Source: three-view drawing plus pictorial views. Frame: mm from the lowest corner of the part. Coordinates: 2 decimals unless noted, no trailing zeros. Write each loop counter-clockwise with the first axis right and the second up, starting at its lowest first coordinate (ties: lowest second). Pieces come first, ordered by that corner, then holes. Notation, with made-up numbers: M 69.25,4.5 L 99.25,4.5 A24 ccw 99.25,26.5 Z; hole C -27,87 d4. An arc over 180 degrees is marked long. Write item = value, one per line. Start each with the question number.
Item 1: Ray query, L1, parallel to X at y = 27, z = 9.5; L2, parallel to X at y = 27.5, z = 20.25 (1 decimal); L3, parallel to X at y = 188, z = 11.25. Return the intervals inside material, ascending. Write a range as [from, to].
Item 2: First-contact query: pin 1 Ø10 at (y, z) = (190.5, 13.5) entering from +X (1 decimal); pin 2 Ø5 at (y, z) = (37, 10) entering from -X; pin 3 Ø20 at (x, y) = (265, 30) entering from +Z; pin 4 Ø8 at (y, z) = (38, 13) entering from +X. Flat tips, straight axial feed; report the tip coordinate or a pass-through.
Item 3: Section C-C on y = 188. Output: boundary loops of the cut face in (x, z).
Item 4: Section B-B on z = 4. Output: boundary loops of the cut face in (x, y) (1 decimal), plus the area to 4 significant figures.
Item 5: Section D-D on x = 177. Output: boundary loops of the cut face in (y, z) (1 decimal), plus the area to 3 significant figures.
Item 6: Section A-A on y = 30. Output: boundary loops of the cut face in (x, z), plus the area to 3 significant figures.
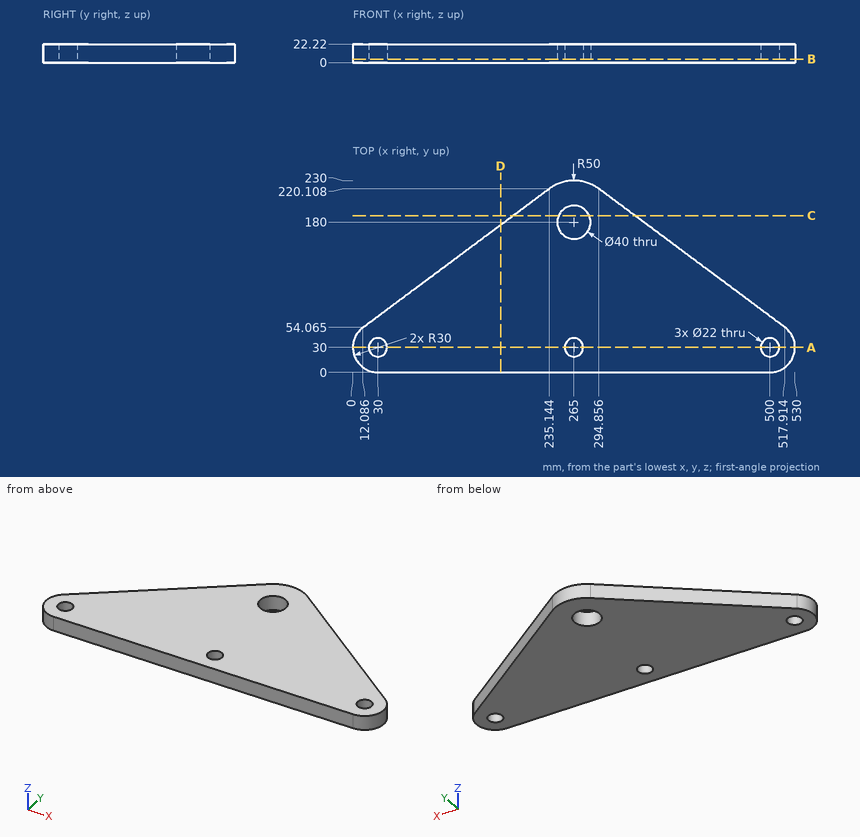
Responses:
q1.L1 = [0.15, 19.42], [40.58, 254.42], [275.58, 489.42], [510.58, 529.85]
q1.L2 = [0.1, 19.3], [40.7, 254.3], [275.7, 489.3], [510.7, 529.9]
q1.L3 = [192.01, 246.67], [283.33, 337.99]
q2.pin_1 = 341.3
q2.pin_2 = 0.34
q2.pin_3 = through
q2.pin_4 = 529.73
q3.outline = M 192.01,0 L 246.67,0 L 246.67,22.22 L 192.01,22.22 Z; M 283.33,0 L 337.99,0 L 337.99,22.22 L 283.33,22.22 Z
q4.outline = M 12.1,54.1 A30 ccw 30,0 L 500,0 A30 ccw 517.9,54.1 L 294.9,220.1 A50 ccw 235.1,220.1 Z; hole C 30,30 d22; hole C 265,180 d40; hole C 265,30 d22; hole C 500,30 d22
q4.area = 73,050 mm²
q5.outline = M 0,0 L 176.8,0 L 176.8,22.2 L 0,22.2 Z
q5.area = 3,930 mm²
q6.outline = M 0,0 L 19,0 L 19,22.22 L 0,22.22 Z; M 41,0 L 254,0 L 254,22.22 L 41,22.22 Z; M 276,0 L 489,0 L 489,22.22 L 276,22.22 Z; M 511,0 L 530,0 L 530,22.22 L 511,22.22 Z
q6.area = 10,300 mm²
